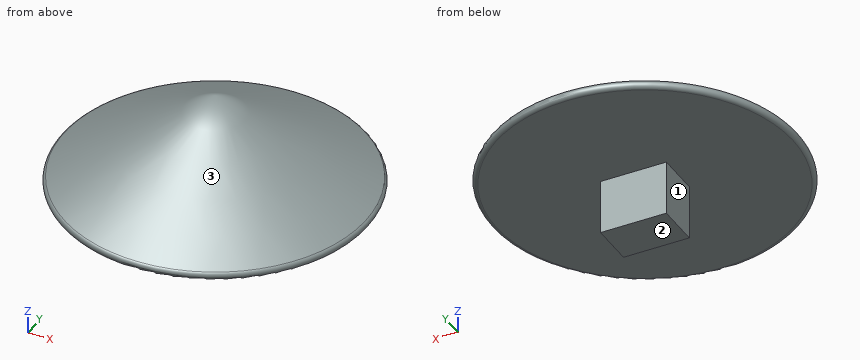
from build123d import *

# Parameters (mm, degrees)
F0_R     = 75
F1_DEPTH = 50
F1_TAPER = 60
F2_W     = 30
F2_H     = 20
F3_DEPTH = 25
F4_R     = 2


with BuildPart() as f1:
    # F0 (on Top) → F1 (new body)
    with BuildSketch(Plane.XY):
        Circle(F0_R)
    extrude(amount=F1_DEPTH, taper=F1_TAPER)

    # F2 (on Top) → F3 (join)
    with BuildSketch(Plane.XY):
        Rectangle(F2_W, F2_H)
    extrude(amount=-F3_DEPTH)

    # F4
    f4_edges = [f1.edges().sort_by_distance(p)[0] for p in [
        (-75, 0, 0),
    ]]
    fillet(f4_edges, radius=F4_R)


solid = f1.part
Part model, mm, in its own coordinate system. Face numbers are marked on the shaded views. Give positions to 0.01 mm unless a question says otherwise; leave off trailing zeros. Write each loop counter-clockwise with the first axis right and the second up, starting at its lowest first coordinate (ties: lowest second). Pieces come first, ordered by that corner, then holes.
1) Cut at B-B on z = 30. Write the cut outline in (x, y), then the cut area to 3 significant figures.
Resolved:
outline: circle Ø46.08 at (0, 0)
area: 1,670 mm2
2) Cut at C-C on z = 11.5. Write the cut outline in (x, y), then the cut area to 3 significant figures.
Resolved:
outline: circle Ø110.16 at (0, 0)
area: 9,530 mm2
3) Cut at A-A on z = -2.5. Write the cut outline in (x, y).
Resolved:
outline: (-15, -10) - (15, -10) - (15, 10) - (-15, 10) - close
4) Pin check, flat tips, straight feed: pin 1 (5 mm diameter, centred on x = -55, y = -13, fed in from +Z); pin 2 (12.5 mm diameter, centred on x = 3.5, z = -14, fed in from -Y); pin 3 (6 mm diameter, centred on y = -1.5, z = -13.5, fed in from -X). Stop position of each tip, or through.
Resolved:
pin 1: stops at z = 12.12
pin 2: stops at y = -10
pin 3: stops at x = -15
5) Two-plate mould, pull along Z, no slides. Class the marked faces 1, 2 and 3: released by +Z, released by -Z, zero draft, split by the parting line, or undercut.
Resolved:
face 1: zero draft
face 2: released by -Z
face 3: released by +Z
6) Probe L1, parallel to X at y = -1.5, z = -13; L2, parallel to Z at x = -13.5, y = -56; L3, parallel to Y at x = -14, z = 31. List the from-to ranges inside material, lowest first.
Resolved:
L1: x = -15 to 15
L2: z = 0 to 10.04
L3: y = -16.06 to 16.06
